For this review, use the dimensioned drawing (mm, ordinates from the lowest corner) and the shaded views. A direction names the side the tool comes from. Coordinates: 2 decimals unless noted, no trailing zeros. Write each loop counter-clockwise with the first axis right and the second up, starting at its lowest first coordinate (ties: lowest second). Pieces come first, ordered by that corner, then holes. Notation, with made-up numbers: M 6,86.25 L 17,86.25 A23 ccw 17,95.25 Z; hole C 87.25,24.5 d2. An arc over 180 degrees is marked long. Return JSON: item names as keys, results as strings.
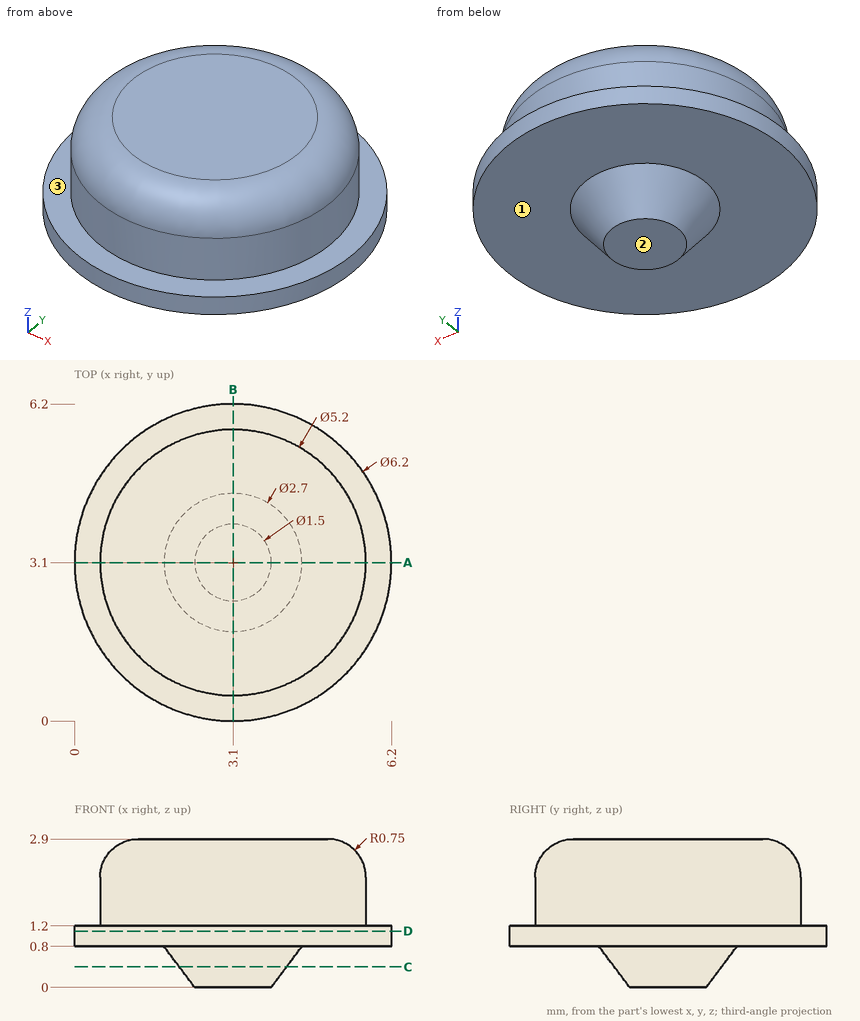
1. Wall thickness on L1, parallel to Z at x = 4.25, y = 4.5; L2, parallel to Z at x = 0.5, y = 2.5; L3, parallel to Y at x = 2.25, z = 2.55: over which ranges is each line inside the solid? List them lowest first. Write a range as from..to.
Checks:
{"L1": "0.8..2.9", "L2": "0.8..1.2", "L3": "0.77..5.43"}
2. Clearance check with flat-ended pins moving along their axes: pin 1 Ø1.5 at (x, z) = (4, 1.5) entering from +Y; pin 2 Ø1 at (y, z) = (1, 2.5) entering from -X. State where each tip first meets the part, or that it passes through.
Checks:
{"pin 1": "y = 6.19", "pin 2": "x = 1.1"}
3. We need section D-D (z = 1.1). State the section outline as (x, y) points.
Checks:
{"outline": "C 3.1,3.1 d6.2"}
4. We need section C-C (z = 0.4). State the section outline as (x, y) points, plus the area to 3 significant figures.
Checks:
{"outline": "C 3.1,3.1 d2.1", "area": "3.46 mm2"}
5. For the marked faces 1, 2 and 3, list the 3-axis set-ups (+Z, -Z, +X, -X, +Y, -Y) from which the entire face can be reached by the end or side of a thin tool; tool diameter is ignored.
Checks:
{"face 1": "-Z", "face 2": "-Z, +X, -X, +Y, -Y", "face 3": "+Z"}
6. We need section A-A (y = 3.1). State the section outline as (x, z) points.
Checks:
{"outline": "M 0,0.8 L 1.75,0.8 L 2.35,0 L 3.85,0 L 4.45,0.8 L 6.2,0.8 L 6.2,1.2 L 5.7,1.2 L 5.7,2.15 A0.75 ccw 4.95,2.9 L 1.25,2.9 A0.75 ccw 0.5,2.15 L 0.5,1.2 L 0,1.2 Z"}
